Check sheet for the modelled part. Datum: model origin and axes. Units: mm. Round coordinates to 2 decimals unless told otherwise and drop trailing zeros. Loops run counter-clockwise (first coordinate to the right, second up) from the corner with the lowest first, then second, coordinate; pieces in that order, holes last. Notation, with made-up numbers: M 48.5,-3.5 L 100.5,-3.5 A28 ccw 100.5,27.5 Z; hole C 5,-32.5 d3. An arc over 180 degrees is marked long. One line per question, with ' | ' between items. Start each with the question number.
(1) Section check A-A (y = -0.75). Record the boundary of the cut face in (x, z).
(2) Go/stop test with flat-tipped pins: P1, Ø1, axis at x = -242, y = -0.5, coming from the +Z side; P2, Ø1, axis at x = -173, y = -2.5, coming from the -Z side. Record where each tip stops, or that it passes through.
(3) Draft check along X on faces 1 (the face through (-388.065, -1.479, 7.828)), 2 (the face through (-2, -3, 8)). Enter one of: +X half, -X half, draft (parallel to the pull), parting line (faces both ways), or undercut.
(4) Thickness scan on probe 1 along X at (y, z) = (-0.9, 7); probe 2 along X at (y, z) = (-2.45, 5); probe 3 along Y at (x, z) = (-146, 2.75). Record the ranges inside material, lowest first. Write a range as [from, to].
(5) Section check B-B (x = -150). Record the boundary of the cut face in (y, z).
```python
from build123d import *

# Parameters (mm, degrees)
F0_W        = 390
F0_H        = 15
F1_DEPTH    = 3
F2_R        = 5
F3_DEPTH    = 20
F4_T1_DEPTH = 405


# Not quite as in the source:
# - a fillet or chamfer that OpenCascade refuses, or shapes differently, is made with other operations: its cross-section is extruded or revolved along the edge and cut away or added


with BuildPart() as f1:
    # F0 (on Front) → F1 (new body)
    with BuildSketch(Plane.XZ):
        with Locations((-195, 7.5)):
            Rectangle(F0_W, F0_H)
    extrude(amount=F1_DEPTH)

    # F2 (on Front) → F3 (cut)
    with BuildSketch(Plane.XZ):
        with Locations((-383.0693596974, 7.6079843566)):
            Circle(F2_R)
        with Locations((-8.0693596974, 7.6553751715)):
            Circle(F2_R)
    extrude(amount=F3_DEPTH, mode=Mode.SUBTRACT)

    # F4: fillet of radius 3 on 4 edges, made by hand

    # F4_s2 → F4_t1 (cut)
    with BuildSketch(Plane.YZ.offset(-397.5)):
        with BuildLine():
            ThreePointArc((-3, 15), (-0.8786796564, 14.1213203436), (0, 12))
            Line((0, 12), (0, 15))
            Line((0, 15), (-3, 15))
        make_face()
        with BuildLine():
            ThreePointArc((0, 3), (-0.8786796564, 0.8786796564), (-3, 0))
            Line((-3, 0), (0, 0))
            Line((0, 0), (0, 3))
        make_face()
        with BuildLine():
            ThreePointArc((0, 15), (-2.1213203436, 14.1213203436), (-3, 12))
            Line((-3, 12), (-3, 15))
            Line((-3, 15), (0, 15))
        make_face()
        with BuildLine():
            ThreePointArc((-3, 3), (-2.1213203436, 0.8786796564), (0, 0))
            Line((0, 0), (-3, 0))
            Line((-3, 0), (-3, 3))
        make_face()
    extrude(amount=F4_T1_DEPTH, mode=Mode.SUBTRACT)


solid = f1.part
```
The answers:
1) outline: M -390,1.02 L 0,1.02 L 0,13.98 L -390,13.98 Z; hole C -383.07,7.61 d10; hole C -8.07,7.66 d10
2) P1: z = 14.24 | P2: z = 0.76
3) face 1: undercut | face 2: draft
4) probe 1: [-390, -388.03], [-378.11, -13.03], [-3.11, 0] | probe 2: [-390, -387.34], [-378.8, -12.31], [-3.83, 0] | probe 3: [-2.99, -0.01]
5) outline: M -3,3 A3 ccw -1.5,0.4 A3 ccw 0,3 L 0,12 A3 ccw -1.5,14.6 A3 ccw -3,12 Z
